from build123d import *

# Parameters (mm, degrees)
SKETCH1_R             = 200
BOSS_EXTRUDE1_DEPTH   = 16
M8_TAPPED_HOLE1_D     = 6.8
CIRPATTERN1_COUNT     = 6
M8X1_0_TAPPED_HOLE1_D = 7


with BuildPart() as part:
    # Sketch1 → Boss-Extrude1 (new body)
    with BuildSketch(Plane(origin=(0, 0, 0), x_dir=(1, 0, 0), z_dir=(0, 1, 0))):
        with Locations(Location((0, 0, 0), (0, 0, 270))):
            Circle(SKETCH1_R)
    extrude(amount=BOSS_EXTRUDE1_DEPTH)

    # M8 Tapped Hole1 (through all)
    with Locations(Plane(origin=(0, 16, 0), x_dir=(1, 0, 0), z_dir=(0, 1, 0))):
        with Locations((0, 25)):
            m8_tapped_hole1 = Hole(M8_TAPPED_HOLE1_D / 2)

    # CirPattern1: M8 Tapped Hole1 ×6 about axis
    cirpattern1_axis = Axis((0, 0, 0), (0, 1, 0))
    for i in range(1, CIRPATTERN1_COUNT):
        add(m8_tapped_hole1.rotate(cirpattern1_axis, i * 360 / CIRPATTERN1_COUNT), mode=Mode.SUBTRACT)

    # M8x1.0 Tapped Hole1 (through all)
    with Locations(Plane(origin=(0, 16, 0), x_dir=(1, 0, 0), z_dir=(0, 1, 0))):
        with Locations((0, 150), (0, -150)):
            Hole(M8X1_0_TAPPED_HOLE1_D / 2)


solid = part.part
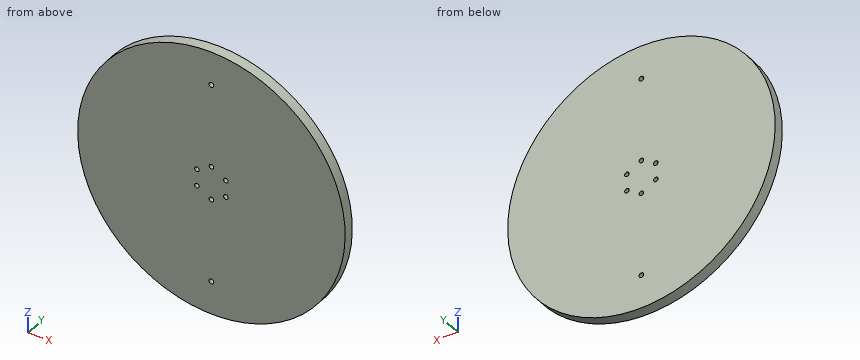
Input: part model. Units: mm. Frame: model coordinates. Give positions to 0.01 mm unless a question says otherwise; leave off trailing zeros. Loops run counter-clockwise (first coordinate to the right, second up) from the corner with the lowest first, then second, coordinate; pieces in that order, holes last. Notation, with made-up numbers: (-1.5, -18.75) - (13.5, -18.75) arc R19 ccw to (13.5, -3.75) - close; hole circle Ø10 at (-13.75, -4.5). An arc over 180 degrees is marked (long way). Use CSV: the item, a comma, the result in double quotes. Start each with the question number.
Item 1: Line query: line 1 (Z direction, x = -0.5, y = 14.75); line 2 (X direction, y = 8.25, z = -1.5); line 3 (X direction, y = 8, z = -150). Output: solid intervals per line, ascending.
Item 2: Section A-A on y = 12. State how many separate pieces and enclosed holes the cut face has, then the cut area to 3 significant figures.
Item 3: Section C-C on z = -109. Return loops of the section in (x, y).
Item 4: Section B-B on x = -103. Return loops of the section in (y, z), then the cut area to 3 significant figures.
Item 5: Contact query for flat-ended pins moving along their axis: P1, Ø4, axis at y = 14, z = 136.5, coming from the -X side; P2, Ø1, axis at x = 70.5, y = 3, coming from the +Z side; P3, Ø4, axis at x = 156, y = 2, coming from the +Z side. Output: stop coordinate, or through.
Ans:
1,line 1,"z = -200 to -153.46, -146.54 to -28.36, -21.64 to 21.64, 28.36 to 146.54, 153.46 to 200"
1,line 2,"x = -199.99 to 199.99"
1,line 3,"x = -132.29 to -3.5, 3.5 to 132.29"
2,separate pieces,"1"
2,enclosed holes,"8"
2,area,"125,000 mm2"
3,outline,"(-167.69, 0) - (167.69, 0) - (167.69, 16) - (-167.69, 16) - close"
4,outline,"(0, -171.44) - (16, -171.44) - (16, 171.44) - (0, 171.44) - close"
4,area,"5,490 mm2"
5,P1,"stops at x = -148.02"
5,P2,"stops at z = 187.35"
5,P3,"stops at z = 127.61"
